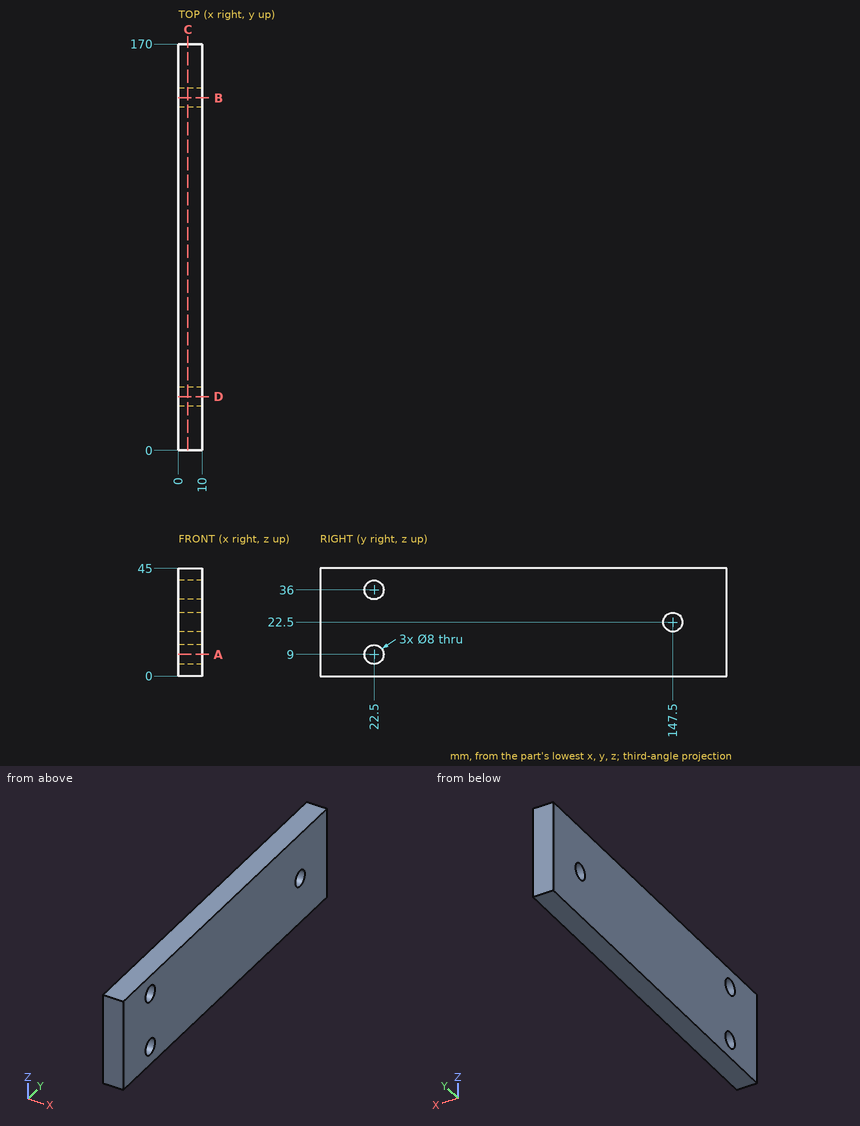
Could you check a few things on this drawing? It's one solid part, dimensions in mm from its lowest x, y, z. Round coordinates to 2 decimals unless told otherwise and drop trailing zeros. Write each loop counter-clockwise with the first axis right and the second up, starting at its lowest first coordinate (ties: lowest second). Pieces come first, ordered by that corner, then holes.
Q1. Please list where these lines run through material, in increasing order: probe 1 along Z at (x, y) = (7.5, 22.5); probe 2 along Z at (x, y) = (3.5, 147.5); probe 3 along Y at (x, z) = (9.25, 8.5).
Q2. If we section it at D-D on y = 22.5: Write out the boundary of the cut face in (x, z), plus the area to 3 significant figures.
Q3. If we section it at B-B on y = 147.5: Write out the boundary of the cut face in (x, z).
Q4. If we section it at C-C on x = 4: Write out the boundary of the cut face in (y, z), plus the area to 3 significant figures.
Q5. If we section it at A-A on z = 9: Write out the boundary of the cut face in (x, y), plus the area to 3 significant figures.
Answer below:
1. probe 1: z = 0 to 5, 13 to 32, 40 to 45
1. probe 2: z = 0 to 18.5, 26.5 to 45
1. probe 3: y = 0 to 18.53, 26.47 to 170
2. outline: (0, 0) - (10, 0) - (10, 5) - (0, 5) - close; (0, 13) - (10, 13) - (10, 32) - (0, 32) - close; (0, 40) - (10, 40) - (10, 45) - (0, 45) - close
2. area: 290 mm2
3. outline: (0, 0) - (10, 0) - (10, 18.5) - (0, 18.5) - close; (0, 26.5) - (10, 26.5) - (10, 45) - (0, 45) - close
4. outline: (0, 0) - (170, 0) - (170, 45) - (0, 45) - close; hole circle Ø8 at (22.5, 9); hole circle Ø8 at (22.5, 36); hole circle Ø8 at (147.5, 22.5)
4. area: 7,500 mm2
5. outline: (0, 0) - (10, 0) - (10, 18.5) - (0, 18.5) - close; (0, 26.5) - (10, 26.5) - (10, 170) - (0, 170) - close
5. area: 1,620 mm2
